For this review, take the finished solid that the model builds, in its own axes (mm). Coordinates: 2 decimals unless noted, no trailing zeros. Write each loop counter-clockwise with the first axis right and the second up, starting at its lowest first coordinate (ties: lowest second). Pieces come first, ordered by that corner, then holes. Notation, with made-up numbers: M 35,42 L 79,42 A18 cw 79,57 Z; hole C 74.25,22.25 d1. An arc over 180 degrees is marked long. One line per question, with ' | ' between items.
from build123d import *

# Parameters (mm, degrees)
SKETCH1_W           = 215
SKETCH1_H           = 113
BOSS_EXTRUDE1_DEPTH = 50
SKETCH2_W           = 110.46
SKETCH2_H           = 48.73
CUT_EXTRUDE1_DEPTH  = 17
SKETCH4_W           = 17
SKETCH4_H           = 80
BOSS_EXTRUDE2_DEPTH = 15
SKETCH6_R           = 1.27
CUT_EXTRUDE4_DEPTH  = 10.16
SKETCH7_W           = 17
SKETCH7_H           = 2.54
CUT_EXTRUDE5_DEPTH  = 8


with BuildPart() as part:
    # Sketch1 → Boss-Extrude1 (new body)
    with BuildSketch(Plane(origin=(0, 0, 0), x_dir=(1, 0, 0), z_dir=(0, 1, 0))):
        with Locations((107.5, 56.5)):
            Rectangle(SKETCH1_W, SKETCH1_H)
    extrude(amount=BOSS_EXTRUDE1_DEPTH)

    # Sketch2 → Cut-Extrude1 (cut)
    with BuildSketch(Plane(origin=(215, 0, 0), x_dir=(0, 0, -1), z_dir=(1, 0, 0))):
        with Locations((56.5, 25.635)):
            Rectangle(SKETCH2_W, SKETCH2_H)
    extrude(amount=-CUT_EXTRUDE1_DEPTH, mode=Mode.SUBTRACT)

    # Sketch4 → Boss-Extrude2 (add)
    with BuildSketch(Plane(origin=(0, 1.27, 0), x_dir=(1, 0, 0), z_dir=(0, 1, 0))):
        with Locations((206.5, 62.73)):
            Rectangle(SKETCH4_W, SKETCH4_H)
    extrude(amount=BOSS_EXTRUDE2_DEPTH)

    # Sketch6 → Cut-Extrude4 (cut)
    with BuildSketch(Plane.XZ):
        with Locations((113.146, -65.278)):
            Circle(SKETCH6_R)
        with Locations((190.87, -65.278)):
            Circle(SKETCH6_R)
    extrude(amount=-CUT_EXTRUDE4_DEPTH, mode=Mode.SUBTRACT)

    # Sketch7 → Cut-Extrude5 (cut)
    with BuildSketch(Plane(origin=(0, 16.27, 0), x_dir=(1, 0, 0), z_dir=(0, 1, 0))):
        with Locations((206.5, 93.84)):
            Rectangle(SKETCH7_W, SKETCH7_H)
        with Locations((206.5, 83.68)):
            Rectangle(SKETCH7_W, SKETCH7_H)
        with Locations((206.5, 73.52)):
            Rectangle(SKETCH7_W, SKETCH7_H)
        with Locations((206.5, 63.36)):
            Rectangle(SKETCH7_W, SKETCH7_H)
        with Locations((206.5, 53.2)):
            Rectangle(SKETCH7_W, SKETCH7_H)
        with Locations((206.5, 43.04)):
            Rectangle(SKETCH7_W, SKETCH7_H)
    extrude(amount=-CUT_EXTRUDE5_DEPTH, mode=Mode.SUBTRACT)


solid = part.part
1) The part is to be moulded in two halves that separate along Z. For faces 1 (the flat face through (215, 8, -60)), 2 (the flat face through (106, 25, 0)), 3 (the flat face through (206, 16.27, -58)), say which applies: +Z half, -Z half, draft (parallel to the pull), parting line (faces both ways), or undercut.
Responses:
face 1: draft | face 2: +Z half | face 3: undercut
2) We need section A-A on y = 38. State the section outline as (x, z) points.
Responses:
outline: M 0,-113 L 215,-113 L 215,-111.73 L 198,-111.73 L 198,-1.27 L 215,-1.27 L 215,0 L 0,0 Z
3) Insertion check: pin 1 Ø14.5 at (y, z) = (33, -37.5) entering from +X; pin 2 Ø6 at (x, z) = (208, -97.5) entering from +Y; pin 3 Ø5 at (x, z) = (207, -17) entering from +Y. Each pin has a flat end and moves straight along its axis. Give the tip position at first contact, or say it passes through.
Responses:
pin 1: x = 198 | pin 2: y = 16.27 | pin 3: y = 1.27
4) To check wall thickness, follow line 1 along Z through (x, y) = (190.87, 5.25); line 2 along X through (y, z) = (25, -82.5); line 3 along Z through (x, y) = (190, 3). State the ranges of each line that lie inside material, in increasing order. Write a range as [from, to].
Responses:
line 1: [-113, -66.55], [-64.01, 0] | line 2: [0, 198] | line 3: [-113, -66.2], [-64.35, 0]
5) We need section B-B on z = -77. State the section outline as (x, y) points.
Responses:
outline: M 0,0 L 215,0 L 215,16.27 L 198,16.27 L 198,50 L 0,50 Z
